Geometry check sheet. Reference: the model listing, model coordinates, mm. A direction names the side the tool comes from. Give positions to 0.01 mm unless a question says otherwise; leave off trailing zeros. Write each loop counter-clockwise with the first axis right and the second up, starting at its lowest first coordinate (ties: lowest second). Pieces come first, ordered by that corner, then holes. Notation, with made-up numbers: M -36,47 L -22,47 A13 ccw -22,71 Z; hole C 77,54.5 d9. An arc over 180 degrees is marked long. One line per item, written item: value. Start each with the question number.
1. Cross-section at C-C on z = 3. Record the cut outline in (x, y), then the cut area to 3 significant figures.
2. Gauge pin test, flat ends, axial feed: pin 1 (2 mm diameter, centred on x = -17, z = 3, fed in from +Y); pin 2 (4.5 mm diameter, centred on x = 17, z = 11, fed in from -Y); pin 3 (1 mm diameter, centred on x = 8.5, y = -4, fed in from -Z); pin 4 (0.8 mm diameter, centred on y = -9, z = 5, fed in from -X). Record the tip position at first contact, or that the pin passes through.
3. Cross-section at A-A on x = 16.25. Record the cut outline in (y, z).
4. Scan lines: line 1 (X direction, y = -7, z = 0.95); line 2 (Z direction, x = 13.85, y = -0.6); line 3 (Y direction, x = -16.25, z = 0.95). Record each from-to range of solid material in increasing order.
5. Tool access check on faces 1 (the face through (-16, -4, 11)), 2 (the face through (-13.814, -5.62, 3.014)), 3 (the face through (12, -4, 6)), 4 (the face through (18.04, -6.96, 2)). Record the directions out of +Z, -Z, +X, -X, +Y, -Y that give a thin tool (end or side, any length) a straight path to the whole face; none if there is none.
6. Cross-section at B-B on z = 10. Record the cut outline in (x, y).
7. Release check for a two-part mould opening along Z. For faces 5 (the face through (15, -5, 0)), 6 (the face through (-12.8, -7.5, 6.1)), 7 (the face through (11.5, -5, 6)) record: pulls with the +Z half, pulls with the -Z half, needs draft (parallel to the pull), parting line crosses it, or undercut.
from build123d import *

# Parameters (mm, degrees)
F1_DEPTH        = 11
F2_W            = 6
F2_H            = 10
F3_DEPTH        = 4
F4_R            = 1.05
F5_DEPTH        = 11
F5_COPIES_COUNT = 2
F5_COPIES_PITCH = 27.7
F7_DEPTH        = 2
F8_R            = 1.6
F9_DEPTH        = 4
F11_DEPTH       = 2


# Not quite as in the source:
# - a pattern or mirror of a feature is missing from the dataset's text; its kind, count and spacing are read off the source's solid


with BuildPart() as f1:
    # F0 (on Front) → F1 (new body)
    with BuildSketch(Plane.XZ):
        Polygon((-19, 4), (-19, 0), (-11.5, 0), (-11.5, 12.5), (11.5, 12.5), (11.5, 0), (19, 0), (19, 4), (13, 4), (13, 14), (-13, 14), (-13, 4), align=None)
    extrude(amount=F1_DEPTH)

    # F2 (on face) → F3 (join)
    with BuildSketch(Plane(origin=(0, 0, 0), x_dir=(-1, 0, 0), z_dir=(0, 1, 0))):
        with Locations((-16, 9)):
            Rectangle(F2_W, F2_H)
        with Locations((16, 9)):
            Rectangle(F2_W, F2_H)
    extrude(amount=-F3_DEPTH)

    # F4 (on Front) → F5 (cut, through all)
    with BuildSketch(Plane.XZ):
        with Locations((-13.85, 6.15)):
            Circle(F4_R)
    f5 = extrude(amount=F5_DEPTH, mode=Mode.SUBTRACT)

    # F5_copies: F5 ×2
    with Locations(*[(i * F5_COPIES_PITCH, 0, 0) for i in range(1, F5_COPIES_COUNT)]):
        add(f5, mode=Mode.SUBTRACT)

    # F6 (on face) → F7 (cut)
    with BuildSketch(Plane.XZ.offset(4)):
        Polygon((-12.6664319482, 8.2), (-15.0335680518, 8.2), (-16.2171361037, 6.15), (-15.0335680518, 4.1), (-12.6664319482, 4.1), (-11.4828638963, 6.15), align=None)
        Polygon((-16.2171361037, 6.15), (-15.0335680518, 8.2), (-19, 8.2), (-19, 4.1), (-15.0335680518, 4.1), align=None)
    f7 = extrude(amount=-F7_DEPTH, mode=Mode.SUBTRACT)

    # F7_copies: F7 across plane
    add(f7.mirror(Plane(origin=(0, 0, 0), x_dir=(0, 0, 1), z_dir=(1, 0, 0))), mode=Mode.SUBTRACT)

    # F8 (on face) → F9 (cut, through all)
    with BuildSketch(Plane(origin=(0, 0, 0), x_dir=(1, 0, 0), z_dir=(0, 0, -1))):
        with Locations((-16.25, 7)):
            Circle(F8_R)
    f9 = extrude(amount=-F9_DEPTH, mode=Mode.SUBTRACT)

    # F9_copies: F9 across plane
    add(f9.mirror(Plane(origin=(0, 0, 0), x_dir=(0, 0, 1), z_dir=(1, 0, 0))), mode=Mode.SUBTRACT)

    # F10 (on face) → F11 (cut)
    with BuildSketch(Plane.XY.offset(4)):
        Polygon((-14.6334192463, -4.2), (-17.8665807537, -4.2), (-19, -6.1631397208), (-19, -7.8368602792), (-17.8665807537, -9.8), (-14.6334192463, -9.8), (-13.0168384925, -7), align=None)
        Polygon((-19, -6.1631397208), (-17.8665807537, -4.2), (-19, -4.2), align=None)
        Polygon((-19, -7.8368602792), (-19, -6.1631397208), (-19.4831615075, -7), align=None)
        Polygon((-17.8665807537, -9.8), (-19, -7.8368602792), (-19, -9.8), align=None)
    f11 = extrude(amount=-F11_DEPTH, mode=Mode.SUBTRACT)

    # F11_copies: F11 across plane
    add(f11.mirror(Plane(origin=(0, 0, 0), x_dir=(0, 0, 1), z_dir=(1, 0, 0))), mode=Mode.SUBTRACT)


solid = f1.part
Report:
1. outline: M -19,-11 L -11.5,-11 L -11.5,0 L -19,0 L -19,-4.2 L -14.63,-4.2 L -13.02,-7 L -14.63,-9.8 L -19,-9.8 Z; M 11.5,-11 L 19,-11 L 19,-9.8 L 14.63,-9.8 L 13.02,-7 L 14.63,-4.2 L 19,-4.2 L 19,0 L 11.5,0 Z
1. area: 107 mm^2
2. pin 1: stops at y = 0
2. pin 2: stops at y = -4
2. pin 3: stops at z = 12.5
2. pin 4: stops at x = -13
3. outline: M -11,0 L -8.6,0 L -8.6,2 L -9.8,2 L -9.8,4 L -11,4 Z; M -5.4,0 L 0,0 L 0,14 L -4,14 L -4,8.2 L -2,8.2 L -2,4.1 L -4,4.1 L -4,4 L -4.2,4 L -4.2,2 L -5.4,2 Z
4. line 1: x = -19 to -17.85, -14.65 to -11.5, 11.5 to 14.65, 17.85 to 19
4. line 2: z = 0 to 5.1, 7.2 to 14
4. line 3: y = -11 to -8.6, -5.4 to 0
5. face 1: +Z, -X, -Y
5. face 2: +Z, -X
5. face 3: +X
5. face 4: +Z, +X
6. outline: M -19,-4 L -13,-4 L -13,-11 L -11.5,-11 L -11.5,0 L -19,0 Z; M 11.5,-11 L 13,-11 L 13,-4 L 19,-4 L 19,0 L 11.5,0 Z
7. face 5: pulls with the -Z half
7. face 6: undercut
7. face 7: needs draft
